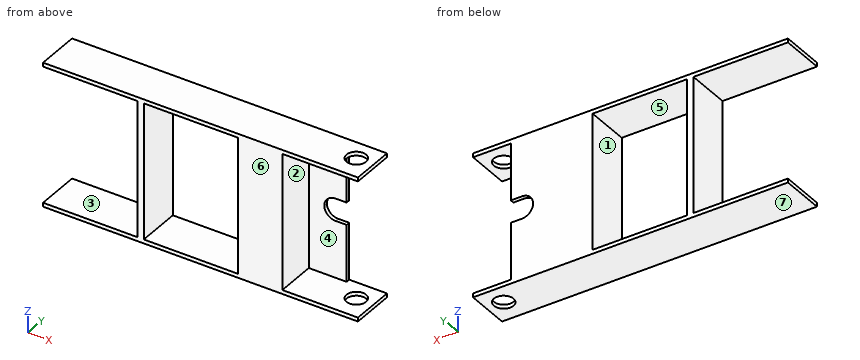
from build123d import *

# Parameters (mm, degrees)
SKETCH1_W               = 127
SKETCH1_H               = 57.9882
BOSS_EXTRUDE1_DEPTH     = 17.70126
SKETCH2_W               = 15.24
SKETCH2_H               = 54.8132
CUT_EXTRUDE1_DEPTH      = 73.015570819
CUT_EXTRUDE2_DEPTH      = 87.756115439
CUT_EXTRUDE2_DEPTH_BACK = 87.756115439
SKETCH3_R               = 3.96875
CUT_EXTRUDE5_DEPTH      = 117.808775528
CUT_EXTRUDE5_DEPTH_BACK = 15.24
SKETCH6_W               = 54.8132
SKETCH6_H               = 16.11376
CUT_EXTRUDE6_DEPTH      = 73.015570819
SKETCH7_W               = 38.1
SKETCH7_H               = 54.8132
CUT_EXTRUDE7_DEPTH      = 73.015570819
SKETCH8_W               = 38.1
SKETCH8_H               = 54.8132
CUT_EXTRUDE8_DEPTH      = 73.015570819


with BuildPart() as part:
    # Sketch1 → Boss-Extrude1 (new body)
    with BuildSketch(Plane(origin=(0, 0, 0), x_dir=(1, 0, 0), z_dir=(0, 1, 0))):
        Rectangle(SKETCH1_W, SKETCH1_H)
    extrude(amount=BOSS_EXTRUDE1_DEPTH)

    # Sketch2 → Cut-Extrude1 (cut, through all)
    with BuildSketch(Plane(origin=(0, 17.70126, 0), x_dir=(1, 0, 0), z_dir=(0, 1, 0))):
        with Locations((55.88, 0)):
            Rectangle(SKETCH2_W, SKETCH2_H)
    extrude(amount=-CUT_EXTRUDE1_DEPTH, mode=Mode.SUBTRACT)

    # Sketch3 → Cut-Extrude2 (cut, two sides: drawn at the far end of the back side and taken through both)
    with BuildSketch(Plane.XY.offset(-27.4066).offset(-CUT_EXTRUDE2_DEPTH_BACK)):
        with Locations((56.515, 9.54786)):
            Circle(SKETCH3_R)
    extrude(amount=CUT_EXTRUDE2_DEPTH + CUT_EXTRUDE2_DEPTH_BACK, mode=Mode.SUBTRACT)

    # Sketch6 → Cut-Extrude5 (cut, two sides: drawn at the far end of the back side and taken through both)
    with BuildSketch(Plane(origin=(48.26, 0, 0), x_dir=(0, 0, -1), z_dir=(1, 0, 0)).offset(-CUT_EXTRUDE5_DEPTH_BACK)):
        with Locations((0, 8.05688)):
            Rectangle(SKETCH6_W, SKETCH6_H)
    extrude(amount=CUT_EXTRUDE5_DEPTH + CUT_EXTRUDE5_DEPTH_BACK, mode=Mode.SUBTRACT)

    # Sketch4 → Cut-Extrude6 (cut, through all)
    with BuildSketch(Plane(origin=(0, 17.70126, 0), x_dir=(1, 0, 0), z_dir=(0, 1, 0))):
        with BuildLine():
            ThreePointArc((43.759999983, 4.500000017), (40.578019456, 3.181980527), (39.259999966, 0))
            Line((39.259999966, 0), (48.26, 0))
            ThreePointArc((48.26, 0), (46.94198051, 3.181980527), (43.759999983, 4.500000017))
        make_face()
        with BuildLine():
            Line((48.26, 0), (39.259999966, 0))
            ThreePointArc((39.259999966, 0), (40.578019456, -3.181980527), (43.759999983, -4.500000017))
            ThreePointArc((43.759999983, -4.500000017), (46.94198051, -3.181980527), (48.26, 0))
        make_face()
        with BuildLine():
            ThreePointArc((43.759999983, 4.500000017), (46.94198051, 3.181980527), (48.26, 0))
            Line((48.26, 0), (48.26, 4.500000017))
            Line((48.26, 4.500000017), (43.759999983, 4.500000017))
        make_face()
        with BuildLine():
            Line((48.26, -4.500000017), (48.26, 0))
            ThreePointArc((48.26, 0), (46.94198051, -3.181980527), (43.759999983, -4.500000017))
            Line((43.759999983, -4.500000017), (48.26, -4.500000017))
        make_face()
    extrude(amount=-CUT_EXTRUDE6_DEPTH, mode=Mode.SUBTRACT)

    # Sketch7 → Cut-Extrude7 (cut, through all)
    with BuildSketch(Plane(origin=(0, 17.70126, 0), x_dir=(1, 0, 0), z_dir=(0, 1, 0))):
        with Locations((-44.45, 0)):
            Rectangle(SKETCH7_W, SKETCH7_H)
    extrude(amount=-CUT_EXTRUDE7_DEPTH, mode=Mode.SUBTRACT)

    # Sketch8 → Cut-Extrude8 (cut, through all)
    with BuildSketch(Plane(origin=(0, 17.70126, 0), x_dir=(1, 0, 0), z_dir=(0, 1, 0))):
        with Locations((-3.81, 0)):
            Rectangle(SKETCH8_W, SKETCH8_H)
    extrude(amount=-CUT_EXTRUDE8_DEPTH, mode=Mode.SUBTRACT)


solid = part.part
Geometry check sheet. Reference: the model listing, model coordinates, mm. Face numbers are marked on the shaded views. A direction names the side the tool comes from. Give positions to 0.01 mm unless a question says otherwise; leave off trailing zeros. Loops run counter-clockwise (first coordinate to the right, second up) from the corner with the lowest first, then second, coordinate; pieces in that order, holes last.
(1) Section check C-C on x = -41. Record the cut outline in (y, z), then the cut area to 3 significant figures.
From the geometry:
outline: (0, -28.99) - (17.7, -28.99) - (17.7, -27.41) - (0, -27.41) - close; (0, 27.41) - (17.7, 27.41) - (17.7, 28.99) - (0, 28.99) - close
area: 56.2 mm2
(2) Depth check by flat-ended pin: pin 1 Ø5 at (y, z) = (15, -20) entering from +X; pin 2 Ø7.5 at (x, z) = (41.5, -11.5) entering from -Y; pin 3 Ø10 at (y, z) = (7.5, 10) entering from +X. Enter the tip coordinate at first touch or a pass-through.
From the geometry:
pin 1: stops at x = 48.26
pin 2: stops at y = 16.11
pin 3: stops at x = 33.02
(3) Section check B-B on z = 23.5. Record the cut outline in (x, y).
From the geometry:
outline: (-25.4, 0) - (-22.86, 0) - (-22.86, 17.7) - (-25.4, 17.7) - close; (15.24, 0) - (33.02, 0) - (33.02, 16.11) - (48.26, 16.11) - (48.26, 17.7) - (15.24, 17.7) - close
(4) Section check A-A on y = 2.75. Record the cut outline in (x, z).
From the geometry:
outline: (-63.5, -28.99) - (63.5, -28.99) - (63.5, -27.41) - (33.02, -27.41) - (33.02, 27.41) - (63.5, 27.41) - (63.5, 28.99) - (-63.5, 28.99) - (-63.5, 27.41) - (-25.4, 27.41) - (-25.4, -27.41) - (-63.5, -27.41) - close; hole (-22.86, -27.41) - (15.24, -27.41) - (15.24, 27.41) - (-22.86, 27.41) - close
(5) Thickness scan on L1, parallel to Z at x = -6.5, y = 3; L2, parallel to X at y = 13, z = -22.5; L3, parallel to Y at x = 43.5, z = 12.5. Record the ranges inside material, lowest first.
From the geometry:
L1: z = -28.99 to -27.41, 27.41 to 28.99
L2: x = -25.4 to -22.86, 15.24 to 33.02
L3: y = 16.11 to 17.7
(6) Set-up check for the marked faces 1, 2 and 3: record each of +Z, -Z, +X, -X, +Y, -Y from which the full face is reachable in a straight line by a thin tool's end or side.
From the geometry:
face 1: +Y, -Y
face 2: +X, -Y
face 3: -X, +Y, -Y
(7) Release check for a two-part mould opening along Z. For the marked faces 4, 5, 6 and 7 record: released by +Z, released by -Z, zero draft, split by the parting line, or undercut.
From the geometry:
face 4: undercut
face 5: undercut
face 6: zero draft
face 7: released by -Z
